Input: part model. Units: mm. Frame: model coordinates. Face numbers are marked on the shaded views. A direction names the side the tool comes from. Round coordinates to 2 decimals unless told otherwise and drop trailing zeros. Order: outer loops, then holes, each group sorted by start corner. A loop starts at its lowest first (then second) coordinate and runs counter-clockwise, first axis right, second up. Notation, with made-up numbers: (-15.5, 30) -> (25.5, 30) arc R28 cw to (25.5, 51) -> close; hole circle Ø4 at (30, -11.75). An arc over 180 degrees is marked (long way). Use a Markdown table: item, result.
Autodesk Inventor part; units mm, degrees
ref_plane "YZ Plane" through (0, 0, 0) normal (1, 0, 0) x (0, 1, 0)
ref_plane "XZ Plane" through (0, 0, 0) normal (0, 1, 0) x (-1, 0, 0)
ref_plane "XY Plane" through (0, 0, 0) normal (0, 0, 1) x (1, 0, 0)
sketch "Sketch1" plane through (0, 0, 0) normal (0, 1, 0) x (-1, 0, 0)
  arc A0 (0, 6.5) -> (0, -6.5) centre (0, 0) ccw
  arc A1 (7.433, 1) -> (6.8739, 3) centre (0, 0) ccw
  line L0 (0, 7.5) -> (-16.5, 7.5)
  line L1 (-16.5, 7.5) -> (-16.5, -7.5)
  line L2 (-16.5, -7.5) -> (0, -7.5)
  line L3 (0, -7.5) -> (0, -6.5)
  line L4 (-16.5, 12.5) -> (-11.5, 12.5)
  line L5 (-11.5, 12.5) -> (-11.5, 7.5)
  line L6 (-11.5, 7.5) -> (-16.5, 7.5)
  line L7 (-16.5, 7.5) -> (-16.5, 12.5)
  line L8 (-16.5, -7.5) -> (-11.5, -7.5)
  line L9 (-11.5, -7.5) -> (-11.5, -12.5)
  line L10 (-11.5, -12.5) -> (-16.5, -12.5)
  line L11 (-16.5, -12.5) -> (-16.5, -7.5)
  line L12 (6.4226, 1) -> (13.4226, 1)
  line L13 (13.4226, 1) -> (13.4226, 3)
  line L14 (13.4226, 3) -> (6.4226, 3)
  line L15 (6.4226, 3) -> (6.4226, 1)
  line L16 (0, 0) -> (-6.5, 0)
  line L17 (6.4226, -1) -> (13.4226, -1)
  line L18 (13.4226, -1) -> (13.4226, -3)
  line L19 (13.4226, -3) -> (6.4226, -3)
  line L20 (6.4226, -3) -> (6.4226, -1)
  arc A2 (7.433, -1) -> (7.5, 0) centre (0, 0) ccw
  arc A3 (6.8739, 3) -> (6.8739, -3) centre (0, 0) ccw
  arc A4 (6.4226, 1) -> (0, 6.5) centre (0, 0) ccw
  arc A5 (7.5, 0) -> (7.433, 1) centre (0, 0) ccw
  arc A6 (6.4226, -1) -> (6.5, 0) centre (0, 0) ccw
  arc A7 (6.8739, -3) -> (7.433, -1) centre (0, 0) ccw
  arc A8 (0, -6.5) -> (5.7663, -3) centre (0, 0) ccw
  line L21 (0, -6.5) -> (0, 6.5)
  line L22 (0, 6.5) -> (0, 7.5)
  arc A9 (5.7663, -3) -> (6.4226, -1) centre (0, 0) ccw
  arc A10 (6.5, 0) -> (6.4226, 1) centre (0, 0) ccw
  dimension "d0" = 13
  dimension "d1" = 15
  dimension "d2" = 15
  dimension "d3" = 16.5
  dimension "d4" = 5
  dimension "d5" = 5
  dimension "d6" = 5
  dimension "d7" = 5
  dimension "d8" = 1
  dimension "d9" = 2
  dimension "d10" = 7
extrude "Extrusion1" add sketch "Sketch1" along normal blind 20 contours L22 A3 L14 L15 A4 | A0 L3 A3 L22 | L15 L14 A1 L12 | A3 L2 L1 L0 | A8 A9 L20 L19 A3 L3 | A1 L14 L13 L12 | L0 L7 L4 L5 | L17 A7 L19 L20 | L9 L10 L11 L2 | A7 L17 L18 L19
sketch "Sketch2" plane through (16.5, 0, 12.5) normal (1, 0, 0) x (0, 0, -1)
  circle A0 centre (22.5, 10) radius 1.5
  line L0 (12.5, 0) -> (12.5, 20)
  line L1 (11.5, 0) -> (11.5, 20)
  line L2 (0, 0) -> (25, 0)
  circle A1 centre (2.5, 10) radius 1.5
  dimension "d13" = 3
  dimension "d14" = 10
  dimension "d15" = 10
extrude "Extrusion2" cut sketch "Sketch2" against normal up to next
sketch "Sketch3" plane through (-13.4226, 0, 3) normal (0, 0, 1) x (1, 0, 0)
  circle A0 centre (2.5488, 10) radius 1.75
  line L0 (6.5488, 20) -> (6.5488, 0)
  line L1 (0, 0) -> (6.5488, 0)
  point P0 (13.4226, 0)
  dimension "d18" = 4
  dimension "d19" = 3.5
  dimension "d20" = 10
extrude "Extrusion3" cut sketch "Sketch3" against normal up to next
sketch "Sketch4" plane through (-6.8739, 0, -3) normal (0, 0, -1) x (-1, 0, 0)
  circle A0 centre (4, 10) radius 1.5
  line L0 (0, 0) -> (0, 20)
  line L1 (0, 0) -> (6.5488, 0)
  point P0 (-6.8739, 0)
  dimension "d23" = 4
  dimension "d24" = 10
  dimension "d25" = 3
extrude "Extrusion4" cut sketch "Sketch4" against normal up to next
properties part number "round_adaptor_13"
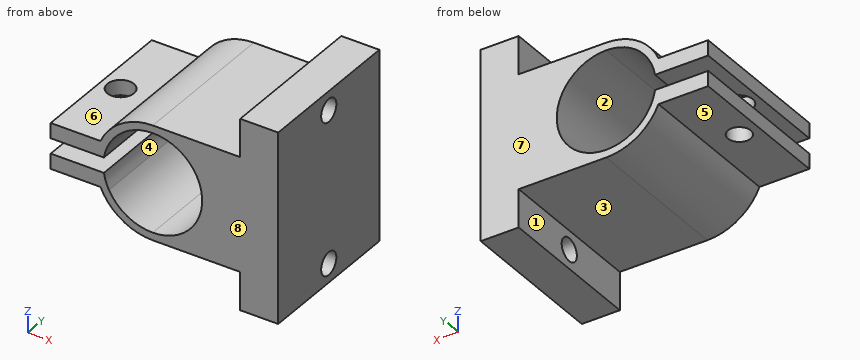
1) Cut plane A-A on z = -2. Return loops of the section in (x, y), and give its area (3 significant figures).
Results found:
| item | result |
|---|---|
| outline | (-13.42, 0) -> (-6.18, 0) -> (-6.18, 20) -> (-13.42, 20) -> close; (6.18, 0) -> (16.5, 0) -> (16.5, 20) -> (6.18, 20) -> close; hole circle Ø3 at (-10.87, 10) |
| area | 344 mm² |
2) Pull-direction query (Z, two-part tool) for the marked faces 1, 2 and 3; classes: +Z half, -Z half, draft (parallel to the pull), parting line (faces both ways), or undercut.
Results found:
| item | result |
|---|---|
| face 1 | draft |
| face 2 | undercut |
| face 3 | -Z half |
3) Set-up query: the marked faces 4, 5, 6, 7 and 8. Return all of +Z, -Z, +X, -X, +Y, -Y with unobstructed straight access to the full face (end or side cutting, diameter ignored); none if empty.
Results found:
| item | result |
|---|---|
| face 4 | +Y, -Y |
| face 5 | -Z, -X, +Y, -Y |
| face 6 | +Z, -X, +Y, -Y |
| face 7 | +Z, -Z, +X, -X, +Y |
| face 8 | +Z, -Z, +X, -X, -Y |
4) Cut plane B-B on x = 12.25. Return loops of the section in (y, z), and give its area (3 significant figures).
Results found:
| item | result |
|---|---|
| outline | (0, -12.5) -> (20, -12.5) -> (20, 12.5) -> (0, 12.5) -> close; hole circle Ø3 at (10, -10); hole circle Ø3 at (10, 10) |
| area | 486 mm² |
5) Line query: L1, parallel to Y at x = 13.55, z = -10; L2, parallel to Z at x = -9, y = 7.5; L3, parallel to Z at x = 9, y = 12.75. Output: solid intervals per line, ascending. Write a range as [from, to].
Results found:
| item | result |
|---|---|
| L1 | y = [0, 8.5], [11.5, 20] |
| L2 | z = [-3, -1], [1, 3] |
| L3 | z = [-7.5, 7.5] |
6) Cut plane C-C on y = 6. Return loops of the section in (x, z), and give its area (3 significant figures).
Results found:
| item | result |
|---|---|
| outline | (-13.42, -3) -> (-6.87, -3) arc R7.5 ccw to (0, -7.5) -> (11.5, -7.5) -> (11.5, -12.5) -> (16.5, -12.5) -> (16.5, 12.5) -> (11.5, 12.5) -> (11.5, 7.5) -> (0, 7.5) arc R7.5 ccw to (-6.87, 3) -> (-13.42, 3) -> (-13.42, 1) -> (-6.42, 1) arc R6.5 cw to (0, 6.5) arc R6.5 cw to (0, -6.5) arc R6.5 cw to (-5.77, -3) arc R6.5 cw to (-6.42, -1) -> (-13.42, -1) -> close |
| area | 276 mm² |
7) Cut plane D-D on z = 10. Return loops of the section in (x, y).
Results found:
| item | result |
|---|---|
| outline | (11.5, 0) -> (16.5, 0) -> (16.5, 8.5) -> (11.5, 8.5) -> close; (11.5, 11.5) -> (16.5, 11.5) -> (16.5, 20) -> (11.5, 20) -> close |
8) Pin query (flat end, axial travel): pin 1 Ø5 at (x, y) = (-9, 15) entering from +Z; pin 2 Ø1.5 at (y, z) = (14, 9.5) entering from -X; pin 3 Ø3 at (x, z) = (-7.5, -6) entering from -Y; pin 4 Ø7.5 at (x, y) = (-9.5, 6.5) entering from -Z. Return the tip coordinate at first contact, or that it passes through.
Results found:
| item | result |
|---|---|
| pin 1 | stops at z = 3.74 |
| pin 2 | stops at x = 11.5 |
| pin 3 | passes through |
| pin 4 | stops at z = -4.82 |
